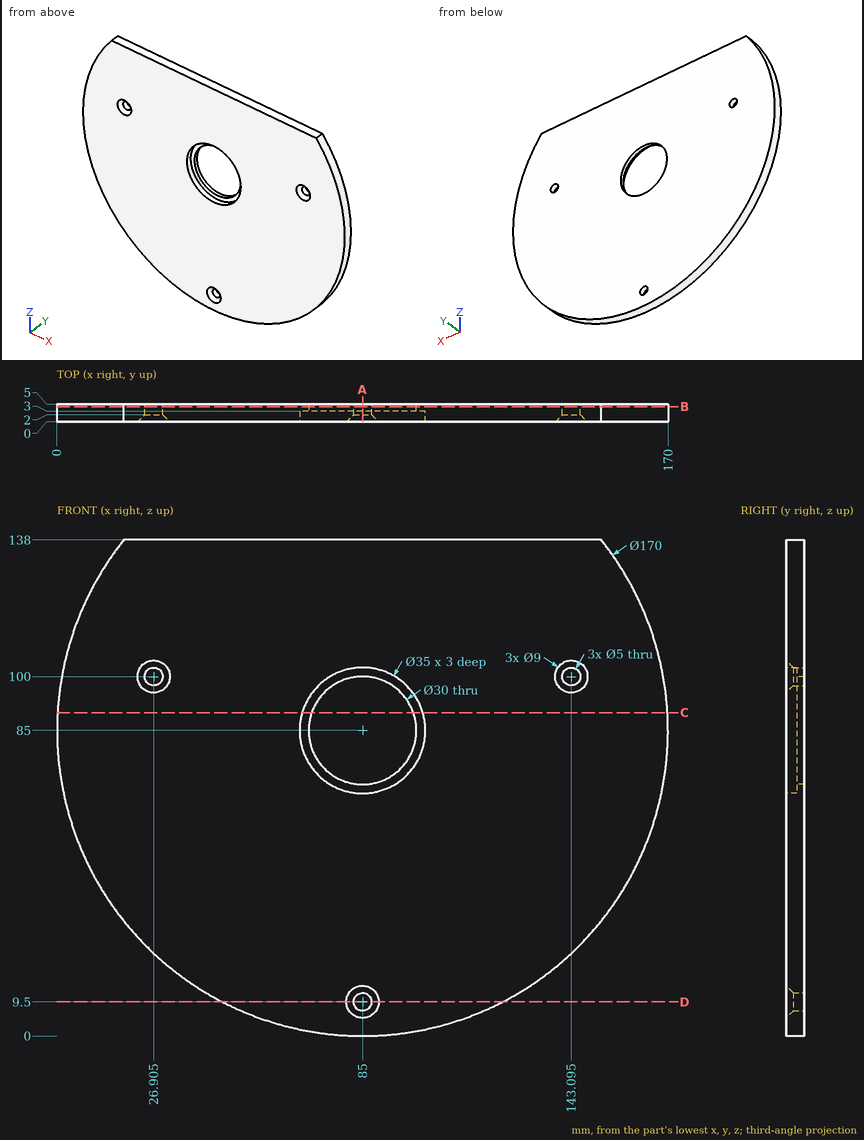
The drawing under review shows one solid part. Ordinate dimensions are in mm from its lowest x, y, z. Give positions to 0.01 mm unless a question says otherwise; leave off trailing zeros. Order: outer loops, then holes, each group sorted by start corner. A loop starts at its lowest first (then second) coordinate and runs counter-clockwise, first axis right, second up. Notation, with made-up numbers: M 29.5,58.5 L 83.5,58.5 A28 cw 83.5,78.5 Z; hole C 47,76.5 d6. An arc over 180 degrees is marked long. Answer in a Markdown table with one row per item. Add a question column.
1. Add section C-C on z = 90. State the section outline as (x, y) points, plus the area to 3 significant figures.
2. Add section A-A on x = 85. State the section outline as (y, z) points, plus the area to 3 significant figures.
3. To check wall thickness, follow line 1 along Z through (x, y) = (85, 2.8); line 2 along X through (y, z) = (1.95, 101); line 3 along X through (y, z) = (2.8, 100) (1 decimal). State the ranges of each line that lie inside material, in increasing order.
4. Add section D-D on z = 9.5. State the section outline as (x, y) points.
5. For pin 1 Ø17.5 at (x, z) = (91, 87.5) entering from -Y; pin 2 Ø1 at (y, z) = (1.5, 73) entering from -X; pin 3 Ø4 at (x, z) = (85, 9.5) entering from -Y; pin 4 Ø1.5 at (x, y) = (35.5, 1.5) entering from -Z, all flat-tipped, find the tip position at first contact; note any pin that passes through.
6. Add section B-B on y = 4.25. State the section outline as (x, z) points (1 decimal).
The answers:
| question | item | result |
|---|---|---|
| 1 | outline | M 0.15,0 L 68.23,0 L 68.23,3 L 70.86,3 L 70.86,5 L 0.15,5 Z; M 99.14,3 L 101.77,3 L 101.77,0 L 169.85,0 L 169.85,5 L 99.14,5 Z |
| 1 | area | 691 mm2 |
| 2 | outline | M 0,0 L 5,0 L 5,7 L 2,7 L 0,5 Z; M 0,14 L 2,12 L 5,12 L 5,70 L 3,70 L 3,67.5 L 0,67.5 Z; M 0,102.5 L 3,102.5 L 3,100 L 5,100 L 5,138 L 0,138 Z |
| 2 | area | 496 mm2 |
| 3 | line 1 | 0 to 7, 12 to 67.5, 102.5 to 138 |
| 3 | line 2 | 1.52 to 24.56, 29.25 to 77.91, 92.09 to 140.75, 145.44 to 168.48 |
| 3 | line 3 | 1.3 to 24.4, 29.4 to 76, 94 to 140.6, 145.6 to 168.7 |
| 4 | outline | M 45.95,0 L 80.5,0 L 82.5,2 L 82.5,5 L 45.95,5 Z; M 87.5,2 L 89.5,0 L 124.05,0 L 124.05,5 L 87.5,5 Z |
| 5 | pin 1 | y = 3 |
| 5 | pin 2 | x = 0.78 |
| 5 | pin 3 | through |
| 5 | pin 4 | z = 15.37 |
| 6 | outline | M 18.5,138 A85 ccw long 151.5,138 Z; hole C 26.9,100 d5; hole C 85,85 d30; hole C 85,9.5 d5; hole C 143.1,100 d5 |
